```python
from build123d import *

# Parameters (mm, degrees)
SKETCH1_W            = 34.29
SKETCH1_H            = 21.59
SKETCH1_R            = 1.7272
BOSS_EXTRUDE1_DEPTH  = 2.54
SKETCH2_W            = 21.59
SKETCH2_H            = 16.256
SKETCH2_R            = 3.8735
BOSS_EXTRUDE2_DEPTH  = 2.54
FILLET1_R            = 5.08
BOSS_EXTRUDE5_DEPTH  = 3.81
MIRROR4_COPY_1_DEPTH = 3.81
FILLET3_R            = 2.54


with BuildPart() as part:
    # Sketch1 → Boss-Extrude1 (new body)
    with BuildSketch(Plane(origin=(0, 0, 0), x_dir=(1, 0, 0), z_dir=(0, 1, 0))):
        Rectangle(SKETCH1_W, SKETCH1_H)
        with Locations(Location((-10, 0, 0), (0, 0, 270))):
            Circle(SKETCH1_R, mode=Mode.SUBTRACT)
        with Locations(Location((10, 0, 0), (0, 0, 270))):
            Circle(SKETCH1_R, mode=Mode.SUBTRACT)
    extrude(amount=BOSS_EXTRUDE1_DEPTH)

    # Sketch2 → Boss-Extrude2 (add)
    with BuildSketch(Plane(origin=(17.145, 0, 0), x_dir=(0, 0, -1), z_dir=(1, 0, 0))):
        with Locations((0, 8.128)):
            Rectangle(SKETCH2_W, SKETCH2_H)
        with Locations((0, 11.176)):
            Circle(SKETCH2_R, mode=Mode.SUBTRACT)
    boss_extrude2 = extrude(amount=BOSS_EXTRUDE2_DEPTH)

    # Mirror1: Boss-Extrude2 across plane
    add(boss_extrude2.mirror(Plane(origin=(0, 0, 0), x_dir=(0, 0, 1), z_dir=(1, 0, 0))))

    # Fillet1
    fillet1_edges = [part.edges().sort_by_distance(p)[0] for p in [
        (-18.415, 16.256, -10.795),
        (-18.415, 16.256, 10.795),
        (18.415, 16.256, 10.795),
        (18.415, 16.256, -10.795),
    ]]
    fillet(fillet1_edges, radius=FILLET1_R)

    # Sketch11 → Boss-Extrude5 (add)
    with BuildSketch(Plane.ZY.offset(19.685)):
        with BuildLine():
            Line((-10.795, 0), (-10.795, -4.437141758))
            ThreePointArc((-10.795, -4.437141758), (-7.088953516, -1.734962797), (-2.75, -0.248344462))
            Line((-2.75, -0.248344462), (-2.75, 0))
            Line((-2.75, 0), (-10.795, 0))
        make_face()
    boss_extrude5 = extrude(amount=-BOSS_EXTRUDE5_DEPTH)

    # Mirror3: Boss-Extrude5 across plane
    add(boss_extrude5.mirror(Plane.XY))

    # Mirror4: Boss-Extrude5 across plane
    add(boss_extrude5.mirror(Plane(origin=(0, 0, 0), x_dir=(0, 0, 1), z_dir=(1, 0, 0))))

    # Mirror4 copy 1 sketch → Mirror4 copy 1 (add)
    with BuildSketch(Plane(origin=(19.685, 0, 0), x_dir=(0, 0, -1), z_dir=(1, 0, 0))):
        with BuildLine():
            Line((-10.795, 0), (-10.795, -4.437141758))
            ThreePointArc((-10.795, -4.437141758), (-7.088953516, -1.734962797), (-2.75, -0.248344462))
            Line((-2.75, -0.248344462), (-2.75, 0))
            Line((-2.75, 0), (-10.795, 0))
        make_face()
    extrude(amount=-MIRROR4_COPY_1_DEPTH)

    # Fillet3
    fillet3_edges = [part.edges().sort_by_distance(p)[0] for p in [
        (-17.145, 2.54, 0),
        (17.145, 2.54, 0),
    ]]
    fillet(fillet3_edges, radius=FILLET3_R)


solid = part.part
```
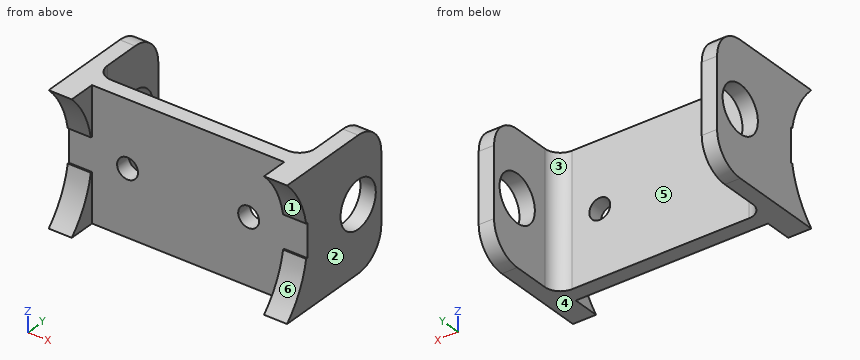
The model under review builds one solid part; all positions refer to its coordinate system, in mm. Face numbers are marked on the shaded views. A direction names the side the tool comes from. Coordinates: 2 decimals unless noted, no trailing zeros. Loops run counter-clockwise (first coordinate to the right, second up) from the corner with the lowest first, then second, coordinate; pieces in that order, holes last. Notation, with made-up numbers: (14, 75) -> (28, 75) arc R23 ccw to (28, 113) -> close; hole circle Ø1 at (19.25, 42.25). An arc over 180 degrees is marked (long way). Answer as CSV lines item,"result".
Item 1: Take a section at B-B, the plane z = 0. State the section outline as (x, y) points (1 decimal), and give its area (3 significant figures).
Results below:
outline,"(-19.7, 0) -> (-11.7, 0) -> (-11.7, 2.5) -> (-14.6, 2.5) arc R2.5 cw to (-17.1, 5.1) -> (-17.1, 7.3) -> (-19.7, 7.3) -> close; (-19.7, 15) -> (-17.1, 15) -> (-17.1, 16.3) -> (-19.7, 16.3) -> close; (-8.3, 0) -> (8.3, 0) -> (8.3, 2.5) -> (-8.3, 2.5) -> close; (11.7, 0) -> (19.7, 0) -> (19.7, 7.3) -> (17.1, 7.3) -> (17.1, 5.1) arc R2.5 cw to (14.6, 2.5) -> (11.7, 2.5) -> close; (17.1, 15) -> (19.7, 15) -> (19.7, 16.3) -> (17.1, 16.3) -> close"
area,"116 mm2"
Item 2: Draft analysis for pull direction X (two halves, no side actions). For the marked faces 1, 2 and 3, state which applies: +X half, -X half, draft (parallel to the pull), parting line (faces both ways), or undercut.
Results below:
face 1,"draft"
face 2,"+X half"
face 3,"undercut"
Item 3: Machinability: for the marked faces 4, 5 and 6, which of the approach directions +Z, -Z, +X, -X, +Y, -Y give a long, thin tool a straight path to every point of the face, cutting with its end or side? Answer none if there is none.
Results below:
face 4,"-Z, +X, -X, +Y, -Y"
face 5,"+Z, -Z, +Y"
face 6,"+X, -X, -Y"
Item 4: Take a section at C-C, the plane x = -10. State the section outline as (y, z) points (3 decimals), and give its area (3 significant figures).
Results below:
outline,"(0, -10.795) -> (2.54, -10.795) -> (2.54, -1.727) -> (0, -1.727) -> close; (0, 1.727) -> (2.54, 1.727) -> (2.54, 10.795) -> (0, 10.795) -> close"
area,"46.1 mm2"
Item 5: For L1, parallel to X at y = 0.95, z = 0 (3 decimals); L2, parallel to Y at x = 17.9, z = 0; L3, parallel to X at y = -2, z = -8.25 (3 decimals), list the stretches that pass through material, from the lowest coordinate up.
Results below:
L1,"x = -19.685 to -11.727, -8.273 to 8.273, 11.727 to 19.685"
L2,"y = 0 to 7.3, 15.05 to 16.26"
L3,"x = -19.685 to -15.875, 15.875 to 19.685"
Item 6: Insertion check: pin 1 (7 mm diameter, centred on y = 11.176, z = 0, fed in from -X); pin 2 (6.5 mm diameter, centred on x = -1.5, z = 3.5, fed in from +Y); pin 3 (2 mm diameter, centred on x = -15, z = -0.5, fed in from -Y). Each pin has a flat end and moves straight along its axis. Give the tip position at first contact, or say it passes through.
Results below:
pin 1,"passes through"
pin 2,"stops at y = 2.54"
pin 3,"stops at y = 0"
Item 7: Take a section at A-A, the plane y = 6. State the section outline as (x, z) points (3 decimals), and give its area (3 significant figures).
Results below:
outline,"(-19.685, -10.795) -> (-17.145, -10.795) -> (-17.145, 10.795) -> (-19.685, 10.795) -> close; (17.145, -10.795) -> (19.685, -10.795) -> (19.685, 10.795) -> (17.145, 10.795) -> close"
area,"110 mm2"
Item 8: Take a section at D-D, the plane y = 8.75. State the section outline as (x, z) points (3 decimals), and give its area (3 significant figures).
Results below:
outline,"(-19.685, -10.795) -> (-17.145, -10.795) -> (-17.145, -3.02) -> (-19.685, -3.02) -> close; (-19.685, 3.02) -> (-17.145, 3.02) -> (-17.145, 10.795) -> (-19.685, 10.795) -> close; (17.145, -10.795) -> (19.685, -10.795) -> (19.685, -3.02) -> (17.145, -3.02) -> close; (17.145, 3.02) -> (19.685, 3.02) -> (19.685, 10.795) -> (17.145, 10.795) -> close"
area,"79.0 mm2"
